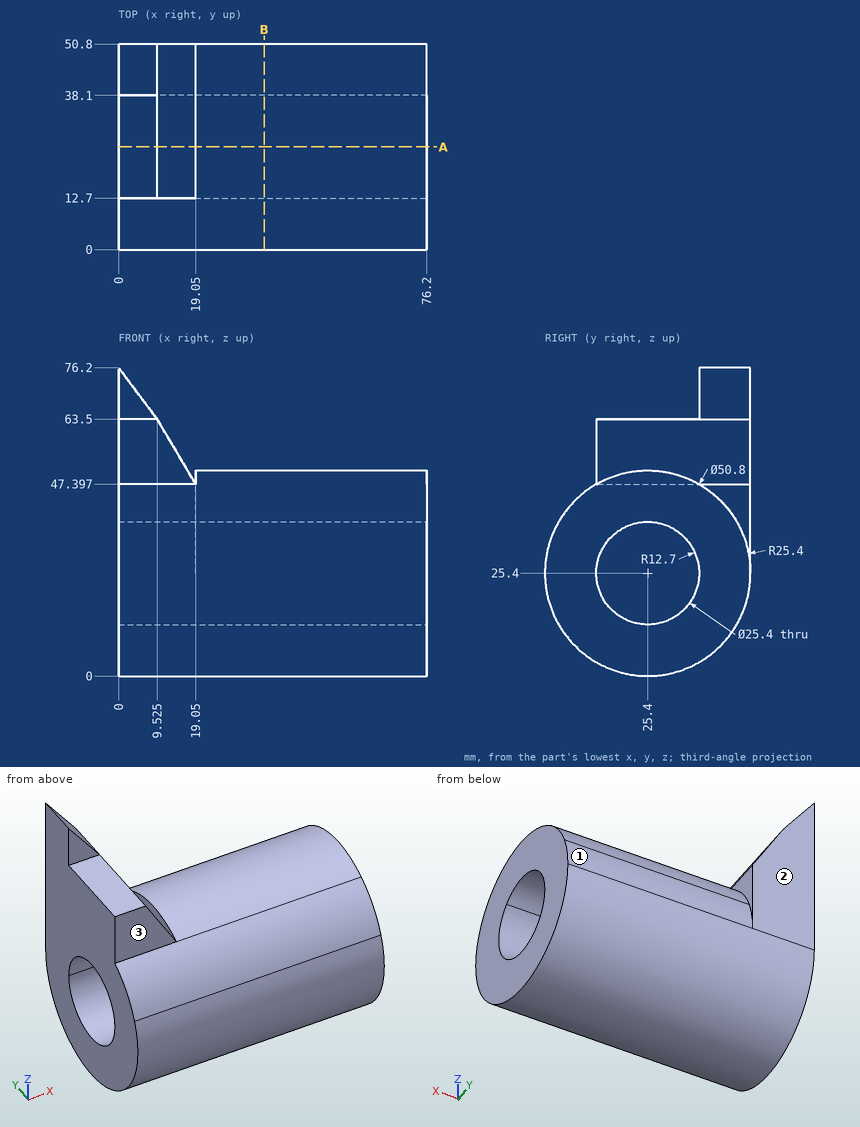
Verification items for this drawing (mm, ordinates from the low corner). A direction names the side the tool comes from. Coordinates: 2 decimals unless noted, no trailing zeros. Loops run counter-clockwise (first coordinate to the right, second up) from the corner with the lowest first, then second, coordinate; pieces in that order, holes last. Notation, with made-up numbers: (-27, 24) - (4, 24) arc R27 ccw to (4, 42) - close; hole circle Ø1 at (69, 57). An arc over 180 degrees is marked (long way). Use one line per item in the form item = value. Start each with the question number.
Item 1: Tool access check on the marked faces 1, 2 and 3. Record the directions out of +Z, -Z, +X, -X, +Y, -Y that give a thin tool (end or side, any length) a straight path to the whole face; none if there is none.
Item 2: Section check B-B, the plane x = 36. Enter the section's corners in (y, z) (1 decimal).
Item 3: Gauge pin test, flat ends, axial feed: pin 1 (12 mm diameter, centred on x = 52.5, y = 20, fed in from +Z); pin 2 (7.5 mm diameter, centred on x = 4.5, z = 69.5, fed in from -Y); pin 3 (3 mm diameter, centred on x = 20.5, z = 19.5, fed in from -Y); pin 4 (1.5 mm diameter, centred on y = 23.5, z = 9.5, fed in from -X). Record the tip position at first contact, or that the pin passes through.
Item 4: Section check A-A, the plane y = 25.4. Enter the section's corners in (x, z) (3 decimals).
Item 5: Thickness scan on probe 1 along Y at (x, z) = (51, 25); probe 2 along Z at (x, y) = (20.5, 25.4); probe 3 along Z at (x, y) = (30.5, 15.5) (1 decimal). Record the ranges inside material, lowest first.
Computed:
q1.face_1 = +Z, +X, +Y
q1.face_2 = +Z, -Z, +X, -X, +Y
q1.face_3 = +Z, +X, -X, -Y
q2.outline = (1.9, 34.9) arc R25.4 ccw (long way) to (50.8, 25.4) arc R25.4 ccw to (48.9, 34.9) arc R25.4 ccw to (12.7, 47.4) arc R25.4 ccw to start; hole (33.8, 34.9) arc R12.7 ccw (long way) to (38.1, 25.4) arc R12.7 ccw to start
q3.pin_1 = 50.8
q3.pin_2 = 38.1
q3.pin_3 = 0.38
q3.pin_4 = 0
q4.outline = (0, 0) - (76.2, 0) - (76.2, 12.7) - (0, 12.7) - close; (0, 38.1) - (76.2, 38.1) - (76.2, 50.8) - (19.05, 50.8) - (19.05, 47.397) - (9.525, 63.5) - (0, 63.5) - close
q5.probe_1 = 0 to 12.71, 38.09 to 50.8
q5.probe_2 = 0 to 12.7, 38.1 to 50.8
q5.probe_3 = 2 to 17.4, 33.4 to 48.8
